Input: dimensioned drawing with shaded views. Units: mm. Origin: part minimum x, y, z. Round coordinates to 2 decimals unless told otherwise and drop trailing zeros. Loops run counter-clockwise (first coordinate to the right, second up) from the corner with the lowest first, then second, coordinate; pieces in that order, holes last. Notation, with made-up numbers: M 15.5,49 L 27.5,49 A32 cw 27.5,82 Z; hole C 83,44 d8. An arc over 180 degrees is marked long. Return JSON: item names as keys, results as strings.
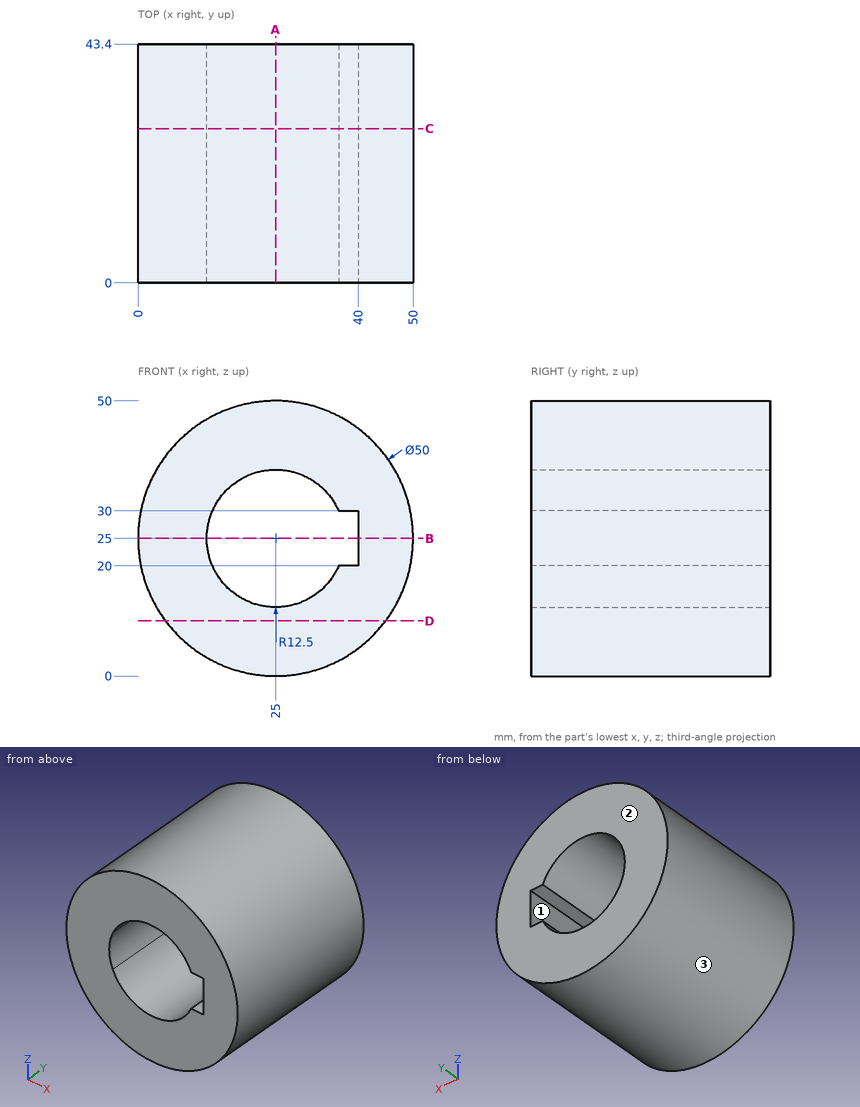
Q1. Pull-direction query (Z, two-part tool) for the marked faces 1, 2 and 3; classes: pulls with the +Z half, pulls with the -Z half, needs draft (parallel to the pull), parting line crosses it, or undercut.
Determined:
{"face 1": "undercut", "face 2": "needs draft", "face 3": "parting line crosses it"}
Q2. Section query A-A (x = 25). Output: boundary loops of the cut face in (y, z).
Determined:
{"outline": "M 0,0 L 43.4,0 L 43.4,12.5 L 0,12.5 Z; M 0,37.5 L 43.4,37.5 L 43.4,50 L 0,50 Z"}
Q3. Section query D-D (z = 10). Output: boundary loops of the cut face in (x, y), plus the area to 3 significant figures.
Determined:
{"outline": "M 5,0 L 45,0 L 45,43.4 L 5,43.4 Z", "area": "1,740 mm^2"}
Q4. Pin query (flat end, axial travel): pin 1 (2 mm diameter, centred on x = 29, y = 14.5, fed in from +Z); pin 2 (8 mm diameter, centred on y = 33.5, z = 11.5, fed in from +X); pin 3 (1.1 mm diameter, centred on x = 39, y = 15, fed in from +Z). Return the tip coordinate at first contact, or that it passes through.
Determined:
{"pin 1": "stops at z = 49.82", "pin 2": "stops at x = 48.12", "pin 3": "stops at z = 46.07"}
Q5. Material intervals for L1, parallel to X at y = 19, z = 18; L2, parallel to X at y = 3.5, z = 13.5; L3, parallel to Z at x = 38, y = 34.5, sorted ascending.
Determined:
{"L1": "x = 1 to 14.64, 35.36 to 49", "L2": "x = 2.8 to 20.1, 29.9 to 47.2", "L3": "z = 3.65 to 20, 30 to 46.35"}
Q6. Section query B-B (z = 25). Output: boundary loops of the cut face in (x, y), plus the area to 4 significant figures.
Determined:
{"outline": "M 0,0 L 12.5,0 L 12.5,43.4 L 0,43.4 Z; M 40,0 L 50,0 L 50,43.4 L 40,43.4 Z", "area": "976.5 mm^2"}
Q7. Section query C-C (y = 28). Output: boundary loops of the cut face in (x, z), plus the area to 3 significant figures.
Determined:
{"outline": "C 25,25 d50; hole M 36.46,20 L 40,20 L 40,30 L 36.46,30 A12.5 ccw long Z", "area": "1,440 mm^2"}
